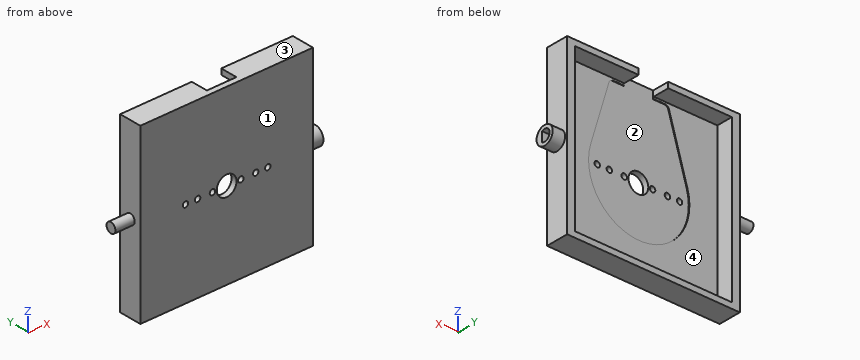
Autodesk Inventor part; units mm, degrees
ref_plane "YZ Plane" through (0, 0, 0) normal (1, 0, 0) x (0, 1, 0)
ref_plane "XZ Plane" through (0, 0, 0) normal (0, 1, 0) x (-1, 0, 0)
ref_plane "XY Plane" through (0, 0, 0) normal (0, 0, 1) x (1, 0, 0)
sketch "Sketch1" plane through (0, 0, 0) normal (0, 1, 0) x (-1, 0, 0)
  line L0 (0, 0) -> (0, 0) construction
  line L1 (-48.26, 48.26) -> (48.26, 48.26)
  line L2 (48.26, 48.26) -> (48.26, -48.26)
  line L3 (48.26, -48.26) -> (-48.26, -48.26)
  line L4 (-48.26, -48.26) -> (-48.26, 48.26)
  line L5 (-48.26, 48.26) -> (48.26, -48.26) construction
  line L6 (48.26, 48.26) -> (-48.26, -48.26) construction
  dimension "d15" = 0
  dimension "d16" = 96.52
extrude "Extrusion2" add sketch "Sketch1" along normal blind 3.556
sketch "Sketch7" plane through (0, 3.556, 0) normal (0, 1, 0) x (1, 0, 0)
  arc A0 (27.0056, -8.0993) -> (-27.0056, -8.0993) centre (0, 0) ccw
  line L0 (0, -43.942) -> (14.366, -43.942)
  line L1 (-14.366, -43.942) -> (0, -43.942)
  line L2 (0, 15.1299) -> (0, -95.843) construction
  line L3 (33.8234, 0) -> (-34.0336, 0) construction
  line L4 (16.256, 0) -> (16.256, -43.942) construction
  line L5 (16.7989, -42.1317) -> (27.0056, -8.0993)
  line L6 (-16.7989, -42.1317) -> (-27.0056, -8.0993)
  circle A1 centre (0, 0) radius 5.5372
  arc A2 (14.366, -43.942) -> (16.7989, -42.1317) centre (14.366, -41.402) ccw
  arc A3 (-16.7989, -42.1317) -> (-14.366, -43.942) centre (-14.366, -41.402) ccw
  circle A4 centre (7.9375, 0) radius 1.524
  line L7 (0, 0) -> (7.9375, 0) construction
  circle A5 centre (-7.9375, 0) radius 1.524
  line L8 (0, 0) -> (-7.9375, 0) construction
  circle A6 centre (16.256, 0) radius 1.524
  line L9 (0, 0) -> (16.256, 0) construction
  circle A7 centre (-16.256, 0) radius 1.524
  line L10 (0, 0) -> (-16.256, 0) construction
  circle A8 centre (23.0124, 0) radius 1.524
  line L11 (0, 0) -> (23.0124, 0) construction
  circle A9 centre (-23.0124, 0) radius 1.524
  line L12 (0, 0) -> (-23.0124, 0) construction
  line L13 (-48.26, -48.26) -> (48.26, -48.26)
  line L14 (8.255, -39.624) -> (-8.255, -39.624)
  line L15 (-8.255, -39.624) -> (-8.255, -48.26)
  line L16 (-8.255, -48.26) -> (8.255, -48.26)
  line L17 (8.255, -48.26) -> (8.255, -39.624)
  line L18 (8.255, -39.624) -> (-8.255, -48.26) construction
  line L19 (-8.255, -39.624) -> (8.255, -48.26) construction
  point P0 (-16.256, -43.942)
  dimension "d43" = 56.388
  dimension "d44" = 16.256
  dimension "d45" = 16.256
  dimension "d46" = 43.942
  dimension "d47" = 11.0744
  dimension "d48" = 2.54
  dimension "d49" = 3.048
  dimension "d50" = 7.9375
  dimension "d51" = 3.048
  dimension "d52" = 16.256
  dimension "d53" = 3.048
  dimension "d54" = 23.0124
  dimension "d77" = 16.51
extrude "Extrusion3" cut sketch "Sketch7" against normal blind 0.381
sketch "Sketch8" plane through (0, 0, 0) normal (0, -1, 0) x (1, 0, 0)
  arc A0 (27.0056, -8.0993) -> (-27.0056, -8.0993) centre (0, 0) ccw
  line L0 (0, -43.942) -> (14.366, -43.942)
  line L1 (-14.366, -43.942) -> (0, -43.942)
  line L2 (0, 15.1299) -> (0, -95.843) construction
  line L3 (33.8234, 0) -> (-34.0336, 0) construction
  line L4 (16.256, 0) -> (16.256, -43.942) construction
  line L5 (16.7989, -42.1317) -> (27.0056, -8.0993)
  line L6 (-16.7989, -42.1317) -> (-27.0056, -8.0993)
  circle A1 centre (0, 0) radius 5.5372
  arc A2 (14.366, -43.942) -> (16.7989, -42.1317) centre (14.366, -41.402) ccw
  arc A3 (-16.7989, -42.1317) -> (-14.366, -43.942) centre (-14.366, -41.402) ccw
  circle A4 centre (7.9375, 0) radius 1.524
  line L7 (0, 0) -> (7.9375, 0) construction
  circle A5 centre (-7.9375, 0) radius 1.524
  line L8 (0, 0) -> (-7.9375, 0) construction
  circle A6 centre (16.256, 0) radius 1.524
  line L9 (0, 0) -> (16.256, 0) construction
  circle A7 centre (-16.256, 0) radius 1.524
  line L10 (0, 0) -> (-16.256, 0) construction
  circle A8 centre (23.0124, 0) radius 1.524
  line L11 (0, 0) -> (23.0124, 0) construction
  circle A9 centre (-23.0124, 0) radius 1.524
  line L12 (0, 0) -> (-23.0124, 0) construction
  point P0 (-16.256, -43.942)
  dimension "d57" = 56.388
  dimension "d58" = 16.256
  dimension "d59" = 16.256
  dimension "d60" = 43.942
  dimension "d61" = 11.0744
  dimension "d62" = 2.54
  dimension "d63" = 3.048
  dimension "d64" = 7.9375
  dimension "d65" = 3.048
  dimension "d66" = 16.256
  dimension "d67" = 3.048
  dimension "d68" = 23.0124
extrude "Extrusion4" cut sketch "Sketch8" against normal blind 3.556 contours A1 | A4 | A5 | A6 | A7 | A8 | A9
sketch "Sketch9" plane through (0, 3.556, 0) normal (0, 1, 0) x (1, 0, 0)
  line L0 (43.815, -45.085) -> (-43.815, -45.085)
  line L1 (-43.815, -45.085) -> (-43.815, 45.085)
  line L2 (-43.815, 45.085) -> (43.815, 45.085)
  line L3 (43.815, 45.085) -> (43.815, -45.085)
  line L4 (43.815, -45.085) -> (-43.815, 45.085) construction
  line L5 (-43.815, -45.085) -> (43.815, 45.085) construction
  line L6 (48.26, -48.26) -> (-48.26, -48.26)
  line L7 (-48.26, -48.26) -> (-48.26, 48.26)
  line L8 (-48.26, 48.26) -> (48.26, 48.26)
  line L9 (48.26, 48.26) -> (48.26, -48.26)
  line L10 (48.26, -48.26) -> (-48.26, 48.26) construction
  line L11 (-48.26, -48.26) -> (48.26, 48.26) construction
  point P0 (0, 0)
  dimension "d71" = 90.17
  dimension "d72" = 87.63
extrude "Extrusion5" add sketch "Sketch9" along normal blind 9.144
sketch "Sketch10" plane through (43.815, 3.556, 45.085) normal (0, 0, -1) x (-1, 0, 0)
  line L0 (0, 9.144) -> (87.63, 9.144)
  line L1 (35.5652, 0) -> (52.0648, 0)
  line L2 (52.0648, 0) -> (52.0648, 9.144)
  line L3 (52.0648, 9.144) -> (35.5652, 9.144)
  line L4 (35.5652, 9.144) -> (35.5652, 0)
  line L5 (35.5652, 0) -> (52.0648, 9.144) construction
  line L6 (52.0648, 0) -> (35.5652, 9.144) construction
  line L7 (43.815, 4.572) -> (87.63, 4.572) construction
  line L8 (43.815, 4.572) -> (0, 4.572) construction
  line L9 (0, 0) -> (0, 9.144) construction
  point P0 (43.815, -3.556)
  dimension "d88" = 28.995
  dimension "d89" = 52.0648
extrude "Extrusion6" cut sketch "Sketch10" against normal up to next
sketch "Sketch14" plane through (-48.26, 0, -48.26) normal (-1, 0, 0) x (0, 0, 1)
  circle A0 centre (48.26, 6.35) radius 2.794
  line L0 (48.26, 6.35) -> (96.52, 6.35) construction
  line L1 (48.26, 6.35) -> (0, 6.35) construction
  line L2 (0, 0) -> (0, 12.7) construction
  point P0 (48.26, 0)
  dimension "d78" = 5.588
  dimension "d90" = 96.52
extrude "Extrusion7" add sketch "Sketch14" along normal blind 10.795
sketch "Sketch15" plane through (48.26, 0, 48.26) normal (1, 0, 0) x (0, 0, -1)
  arc A0 (50.9865, 4.7231) -> (45.5335, 4.7231) centre (48.26, 6.35) ccw
  circle A1 centre (48.26, 6.35) radius 5.08
  line L0 (45.5335, 4.7231) -> (50.9865, 4.7231)
  line L1 (48.26, 6.35) -> (0, 6.35) construction
  line L2 (0, 0) -> (0, 12.7) construction
  line L3 (48.26, 6.35) -> (96.52, 6.35) construction
  line L4 (96.52, 0) -> (96.52, 12.7) construction
  dimension "d81" = 6.35
  dimension "d82" = 10.16
  dimension "d91" = 1.6269
extrude "Extrusion9" add sketch "Sketch15" along normal blind 6.985
properties part number "joystick_inner1"
The listing builds one solid part. Answer for the finished solid, in the listing's coordinates (mm). Face numbers are marked on the shaded views. Coordinates: 2 decimals unless noted, no trailing zeros. Order: outer loops, then holes, each group sorted by start corner. A loop starts at its lowest first (then second) coordinate and runs counter-clockwise, first axis right, second up. Notation, with made-up numbers: M 84,13.25 L 133,13.25 A32 cw 133,46.25 Z; hole C 3.5,45 d5. An arc over 180 degrees is marked long. Answer as a JSON object with one key per item and string values. Group by question number.
1. Determine the mould class of the marked faces 1, 2, 3 and 4 for opening direction Z: released by +Z, released by -Z, zero draft, split by the parting line, or undercut.
2. Straight lines are drawn through the part: line 1 (X direction, y = 4.75, z = -3) (3 decimals); line 2 (X direction, y = 9.25, z = 5) (3 decimals); line 3 (Z direction, x = 33.5, y = 9) (3 decimals). For each, find the intervals that lie inside material, in ascending order.
3. Section C-C on y = 6.35 is taken. Write down the section's boundary in (x, z) (3 decimals), then the cut area to 3 significant figures.
4. Flat-ended cylindrical pins translate along their axes: P1, Ø4, axis at y = 5, z = 22, coming from the -X side; P2, Ø3.5, axis at y = 6, z = 46, coming from the +X side; P3, Ø10, axis at x = 0, z = 0, coming from the -Y side; P4, Ø5, axis at x = -23.01, z = 0, coming from the +Y side (3 decimals). Find the tip coordinate at first contact, or state that the pin passes through.
5. Section A-A on x = 0 is taken. Write down the section's boundary in (y, z) (3 decimals).
6. Section D-D on x = 20 is taken. Write down the section's boundary in (y, z) (3 decimals).
7. Section B-B on z = -42 is taken. Write down the section's boundary in (x, y) (3 decimals).
Values follow:
{
 "1": {"face 1": "zero draft", "face 2": "undercut", "face 3": "released by +Z", "face 4": "undercut"},
 "2": {"line 1": "-48.26 to -43.815, 43.815 to 55.245", "line 2": "-48.26 to -43.815, 43.815 to 48.26", "line 3": "-48.26 to -45.085, 45.085 to 48.26"},
 "3": {"outline": "M -59.055,-2.794 L -48.26,-2.794 L -48.26,-48.26 L 48.26,-48.26 L 48.26,-5.08 L 55.245,-5.08 L 55.245,-3.175 L 48.26,-3.175 L 48.26,3.175 L 55.245,3.175 L 55.245,5.08 L 48.26,5.08 L 48.26,48.26 L 8.25,48.26 L 8.25,45.085 L 43.815,45.085 L 43.815,-45.085 L -43.815,-45.085 L -43.815,45.085 L -8.25,45.085 L -8.25,48.26 L -48.26,48.26 L -48.26,2.794 L -59.055,2.794 Z", "area": "1,450 mm2"},
 "4": {"P1": "x = -48.26", "P2": "x = 48.26", "P3": "through", "P4": "y = 3.175"},
 "5": {"outline": "M 0,-48.26 L 12.7,-48.26 L 12.7,-45.085 L 3.556,-45.085 L 3.556,-28.194 L 3.175,-28.194 L 3.175,-5.537 L 0,-5.537 Z; M 0,5.537 L 3.175,5.537 L 3.175,48.26 L 0,48.26 Z"},
 "6": {"outline": "M 0,-48.26 L 12.7,-48.26 L 12.7,-45.085 L 3.556,-45.085 L 3.556,-19.872 L 3.175,-19.872 L 3.175,31.458 L 3.556,31.458 L 3.556,45.085 L 12.7,45.085 L 12.7,48.26 L 0,48.26 Z"},
 "7": {"outline": "M -48.26,0 L 48.26,0 L 48.26,12.7 L 43.815,12.7 L 43.815,3.556 L -43.815,3.556 L -43.815,12.7 L -48.26,12.7 Z"}
}
